Input: part model. Units: mm. Frame: model coordinates. Coordinates: 2 decimals unless noted, no trailing zeros. Write each loop counter-clockwise with the first axis right and the second up, starting at its lowest first coordinate (ties: lowest second). Pieces come first, ordered by that corner, then holes. Notation, with made-up numbers: (57.5, 47) - (85.5, 47) arc R30 ccw to (85.5, 85) - close; hole circle Ø3 at (80.5, 87). An arc over 180 degrees is marked (long way). Use a Markdown table: item, result. Add a question column.
Q1. Section query B-B (x = 5.75). Return the cut outline in (y, z).
Q2. Section query C-C (z = 0.8). Return the cut outline in (x, y).
Q3. Pin query (flat end, axial travel): P1, Ø2.5, axis at x = -5, y = 5, coming from the +Z side; P2, Ø1.6, axis at x = 5, y = 5, coming from the -Z side. Return the tip coordinate at first contact, or that it passes through.
Q4. Section query D-D (x = -5). Return the cut outline in (y, z).
Q5. Material intervals for probe 1 along Y at (x, z) = (5, 0.7); probe 2 along X at (y, z) = (5.25, 0.5); probe 3 along Y at (x, z) = (5.75, 0.65), sorted ascending. Write a range as from..to.
Q6. Mould query, pull axis Y, two halves, no side actions, for faces 1 (the face through (10, 4.9, 0.5)), 2 (the face through (4.87, 5.99, 0.49)), 3 (the face through (0.4, 0, 0.5)), 4 (the face through (-5.13, 5.99, 0.49)). Classes: released by +Y, released by -Y, zero draft, split by the parting line, or undercut.
Q7. Section query A-A (y = 5). Return the cut outline in (x, z).
from build123d import *

# Parameters (mm, degrees)
SKETCH6_R           = 1
BOSS_EXTRUDE4_DEPTH = 1


with BuildPart() as part:
    # Sketch6 → Boss-Extrude4 (new body)
    with BuildSketch(Plane.XY):
        with BuildLine():
            Line((0, 10), (-3, 10))
            Line((-3, 10), (-4, 10))
            ThreePointArc((-4, 10), (-8.099019514, 5), (-4, 0))
            Line((-4, 0), (-3, 0))
            Line((-3, 0), (0, 0))
            Line((0, 0), (5, 0))
            ThreePointArc((5, 0), (10, 5), (5, 10))
            Line((5, 10), (0, 10))
        make_face()
        with Locations((5, 5)):
            Circle(SKETCH6_R, mode=Mode.SUBTRACT)
        with Locations((-5, 5)):
            Circle(SKETCH6_R, mode=Mode.SUBTRACT)
    extrude(amount=BOSS_EXTRUDE4_DEPTH)


solid = part.part
Values follow:
| question | item | result |
|---|---|---|
| 1 | outline | (0.06, 0) - (4.34, 0) - (4.34, 1) - (0.06, 1) - close; (5.66, 0) - (9.94, 0) - (9.94, 1) - (5.66, 1) - close |
| 2 | outline | (-4, 0) - (5, 0) arc R5 ccw to (5, 10) - (-4, 10) arc R5.1 ccw to start; hole circle Ø2 at (-5, 5); hole circle Ø2 at (5, 5) |
| 3 | P1 | z = 1 |
| 3 | P2 | through |
| 4 | outline | (0.31, 0) - (4, 0) - (4, 1) - (0.31, 1) - close; (6, 0) - (9.69, 0) - (9.69, 1) - (6, 1) - close |
| 5 | probe 1 | 0..4, 6..10 |
| 5 | probe 2 | -8.09..-5.97, -4.03..4.03, 5.97..9.99 |
| 5 | probe 3 | 0.06..4.34, 5.66..9.94 |
| 6 | face 1 | split by the parting line |
| 6 | face 2 | undercut |
| 6 | face 3 | released by -Y |
| 6 | face 4 | undercut |
| 7 | outline | (-8.1, 0) - (-6, 0) - (-6, 1) - (-8.1, 1) - close; (-4, 0) - (4, 0) - (4, 1) - (-4, 1) - close; (6, 0) - (10, 0) - (10, 1) - (6, 1) - close |
